CAD build for the part. Positions are in the model's coordinates, mm. A direction names the side the tool comes from. Give positions to 0.01 mm unless a question says otherwise; leave off trailing zeros. Loops run counter-clockwise (first coordinate to the right, second up) from the corner with the lowest first, then second, coordinate; pieces in that order, holes last. Notation, with made-up numbers: M 84.5,-9.5 L 114.5,-9.5 A27 cw 114.5,19.5 Z; hole C 86,0.25 d7. An arc over 180 degrees is marked long. Answer as CSV lines item,"result".
from build123d import *

# Parameters (mm, degrees)
F0_R     = 44.45
F0_R_2   = 19.05
F1_DEPTH = 6.35
F2_R     = 36.5125
F2_R_2   = 31.75
F3_DEPTH = 76.2
F5_DEPTH = 6.35
F6_W     = 6.35
F6_H     = 50.8
F7_DEPTH = 76.2


with BuildPart() as f1:
    # F0 (on Front) → F1 (new body)
    with BuildSketch(Plane.XZ):
        Circle(F0_R)
        Circle(F0_R_2, mode=Mode.SUBTRACT)
    extrude(amount=F1_DEPTH)

    # F2 (on face) → F3 (join)
    with BuildSketch(Plane.XZ.offset(6.35)):
        Circle(F2_R)
        Circle(F2_R_2, mode=Mode.SUBTRACT)
    extrude(amount=F3_DEPTH)

    # F4 (on face) → F5 (join)
    with BuildSketch(Plane.XZ.offset(82.55)):
        with BuildLine():
            ThreePointArc((0, -44.45), (31.4308964237, -31.4308964237), (44.45, 0))
            ThreePointArc((44.45, 0), (31.4308964237, 31.4308964237), (0, 44.45))
            Line((0, 44.45), (0, 4.7625))
            ThreePointArc((0, 4.7625), (3.3675960454, 3.3675960454), (4.7625, 0))
            ThreePointArc((4.7625, 0), (3.3675960454, -3.3675960454), (0, -4.7625))
            Line((0, -4.7625), (0, -44.45))
        make_face()
        with BuildLine():
            Line((0, 4.7625), (0, 44.45))
            ThreePointArc((0, 44.45), (-44.45, 0), (0, -44.45))
            Line((0, -44.45), (0, -4.7625))
            ThreePointArc((0, -4.7625), (-4.7625, 0), (0, 4.7625))
        make_face()
        with BuildLine():
            ThreePointArc((0, -44.45), (-44.45, 0), (0, 44.45))
            Line((0, 44.45), (-50.8, 44.45))
            Line((-50.8, 44.45), (-50.8, -44.45))
            Line((-50.8, -44.45), (0, -44.45))
        make_face()
    extrude(amount=F5_DEPTH)


with BuildPart() as f7:
    # F6 (on face) → F7 (new body)
    with BuildSketch(Plane.XZ.offset(88.9)):
        with Locations((41.275, 0)):
            Rectangle(F6_W, F6_H)
    extrude(amount=F7_DEPTH)


solid = f1.part
1) Flat gauge pins, fed straight in: pin 1 (12 mm diameter, centred on x = -13, y = -17.5, fed in from -Z); pin 2 (8.5 mm diameter, centred on x = 0, z = 0, fed in from -Y); pin 3 (6 mm diameter, centred on x = -1.5, z = 13.5, fed in from +Y); pin 4 (2 mm diameter, centred on y = -65.5, z = -8.5, fed in from -X). Where does each tip first touch, or does it go through?
Answer below:
pin 1,"stops at z = -35.84"
pin 2,"passes through"
pin 3,"stops at y = -82.55"
pin 4,"stops at x = -35.73"
2) Band-saw the part on B-B on z = 7. Give the cut face in (x, y).
Answer below:
outline,"M -50.8,-88.9 L 43.9,-88.9 L 43.9,-82.55 L 35.84,-82.55 L 35.84,-6.35 L 43.9,-6.35 L 43.9,0 L 17.72,0 L 17.72,-6.35 L 30.97,-6.35 L 30.97,-82.55 L -30.97,-82.55 L -30.97,-6.35 L -17.72,-6.35 L -17.72,0 L -43.9,0 L -43.9,-6.35 L -35.84,-6.35 L -35.84,-82.55 L -50.8,-82.55 Z"
3) Which spindle directions (+Z, -Z, +X, -X, +Y, -Y) get a long thin tool onto all of the face, cutting with end or side? Do faces 5 (the face through (-50.8, -86, 1)), 6 (the face through (-6.883, -43.917, -30.995)), 7 (the face through (-15.12, -3.13, -11.59)). Say none if no direction does.
Answer below:
face 5,"+Z, -Z, -X, +Y, -Y"
face 6,"none"
face 7,"+Y"
4) Band-saw the part on D-D on x = 15.5. Give the cut face in (y, z), and give its area (3 significant figures).
Answer below:
outline,"M -88.9,-41.66 L -82.55,-41.66 L -82.55,-33.06 L -6.35,-33.06 L -6.35,-41.66 L 0,-41.66 L 0,-11.07 L -6.35,-11.07 L -6.35,-27.71 L -82.55,-27.71 L -82.55,27.71 L -6.35,27.71 L -6.35,11.07 L 0,11.07 L 0,41.66 L -6.35,41.66 L -6.35,33.06 L -82.55,33.06 L -82.55,41.66 L -88.9,41.66 Z"
area,"1,730 mm^2"
5) Band-saw the part on A-A on x = 2.5. Give the cut face in (y, z).
Answer below:
outline,"M -88.9,-44.38 L -82.55,-44.38 L -82.55,-36.43 L -6.35,-36.43 L -6.35,-44.38 L 0,-44.38 L 0,-18.89 L -6.35,-18.89 L -6.35,-31.65 L -82.55,-31.65 L -82.55,-4.05 L -88.9,-4.05 Z; M -88.9,4.05 L -82.55,4.05 L -82.55,31.65 L -6.35,31.65 L -6.35,18.89 L 0,18.89 L 0,44.38 L -6.35,44.38 L -6.35,36.43 L -82.55,36.43 L -82.55,44.38 L -88.9,44.38 Z"
6) Drill centre lines: line 1 (Y direction, x = -26, z = 27); line 2 (Z direction, x = 0, y = -29); line 3 (Z direction, x = 0, y = -4). Where is each one in solid material? Low to high. Write a range as from..to.
Answer below:
line 1,"y = -88.9..-82.55, -6.35..0"
line 2,"z = -36.51..-31.75, 31.75..36.51"
line 3,"z = -44.45..-19.05, 19.05..44.45"
7) Mould opens along Y. For faces 1 (the face through (42.397, -3.131, 13.352)), 2 (the face through (9, 0, -19)), 3 (the face through (-14, -88.9, 1)), 4 (the face through (-7, -6.35, 36)) say: +Y half, -Y half, draft (parallel to the pull), parting line (faces both ways), or undercut.
Answer below:
face 1,"draft"
face 2,"+Y half"
face 3,"-Y half"
face 4,"undercut"
